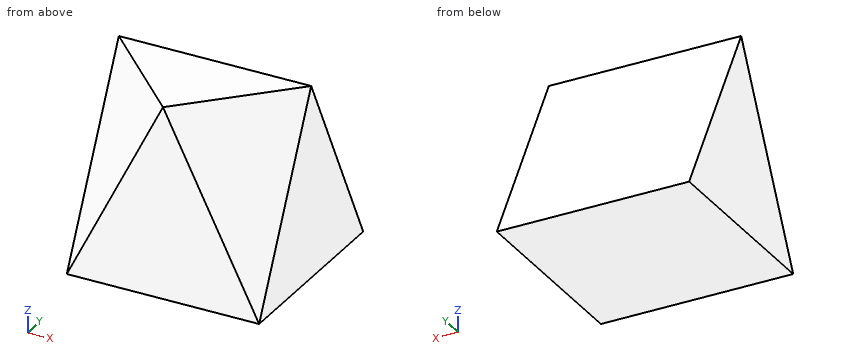
```python
from build123d import *

# Parameters (mm, degrees)
F1_DEPTH = 20
F5_DEPTH = 13.3343333333


# Not quite as in the source:
# - a pattern or mirror of a feature is missing from the dataset's text; its kind, count and spacing are read off the source's solid


with BuildPart() as f1:
    # F0 (on Right) → F1 (new body, symmetric)
    with BuildSketch(Plane.YZ):
        Polygon((0, 40), (0, 0), (40, 0), (20, 40), align=None)
    extrude(amount=F1_DEPTH, both=True)

    # F4 (on 3pt) → F5 (cut, through all)
    with BuildSketch(Plane(origin=(8.8888888889, -8.8888888889, 4.4444444444), x_dir=(-0.7453559925, -0.596284794, 0.298142397), z_dir=(-0.6666666667, 0.6666666667, -0.3333333333))):
        Polygon((-14.90711985, 0), (11.92569588, 35.77708764), (-14.90711985, 44.72135955), align=None)
    f5 = extrude(amount=-F5_DEPTH, mode=Mode.SUBTRACT)

    # F5_copies: F5 across plane
    add(f5.mirror(Plane(origin=(0, 0, 0), x_dir=(0, 0, -1), z_dir=(-1, 0, 0))), mode=Mode.SUBTRACT)


solid = f1.part
```
Geometry: final body of the model. Coordinates: model frame, mm. Round coordinates to 2 decimals unless told otherwise and drop trailing zeros. Loops run counter-clockwise (first coordinate to the right, second up) from the corner with the lowest first, then second, coordinate; pieces in that order, holes last. Notation, with made-up numbers: (-38, 32) -> (-22, 32) arc R20 cw to (-22, 48) -> close; hole circle Ø10 at (34, -5.5). An arc over 180 degrees is marked (long way). Use one line per item in the form item = value.
Item 1: Cut plane A-A on x = 10. Output: boundary loops of the cut face in (y, z), then the cut area to 3 significant figures.
Evaluation:
outline = (0, 0) -> (40, 0) -> (20, 40) -> (10, 40) -> (0, 20) -> close
area = 1,100 mm2
Item 2: Material intervals for probe 1 along X at (y, z) = (2, 17.5); probe 2 along Y at (x, z) = (-4, 26.5); probe 3 along Z at (x, y) = (18, 22), sorted ascending.
Evaluation:
probe_1 = -13.25 to 13.25
probe_2 = 0 to 26.75
probe_3 = 0 to 36
Item 3: Cut plane C-C on y = 16.5. Output: boundary loops of the cut face in (x, z).
Evaluation:
outline = (-20, 0) -> (20, 0) -> (20, 33) -> (16.5, 40) -> (-16.5, 40) -> (-20, 33) -> close
Item 4: Cut plane D-D on x = -7. Output: boundary loops of the cut face in (y, z).
Evaluation:
outline = (0, 0) -> (40, 0) -> (20, 40) -> (7, 40) -> (0, 26) -> close
Item 5: Contact query for flat-ended pins moving along their axis: pin 1 Ø8 at (y, z) = (12.5, 35.5) entering from +X; pin 2 Ø1.5 at (y, z) = (5, 17) entering from -X. Output: stop coordinate, or through.
Evaluation:
pin_1 = 19.22
pin_2 = -17.34
Item 6: Cut plane B-B on z = 37. Output: boundary loops of the cut face in (x, y), then the cut area to 3 significant figures.
Evaluation:
outline = (-20, 18.5) -> (-1.5, 0) -> (1.5, 0) -> (20, 18.5) -> (20, 21.5) -> (-20, 21.5) -> close
area = 518 mm2
